Input: dimensioned drawing with shaded views. Units: mm. Origin: part minimum x, y, z. Give positions to 0.01 mm unless a question says otherwise; leave off trailing zeros. Write each loop counter-clockwise with the first axis right and the second up, starting at its lowest first coordinate (ties: lowest second). Pieces come first, ordered by that corner, then holes. Notation, with made-up numbers: M -37,-12.75 L -4,-12.75 A25 ccw -4,26.25 Z; hole C 18,2 d9. An arc over 180 degrees is marked long. Answer as a JSON object with one key per item and string values.
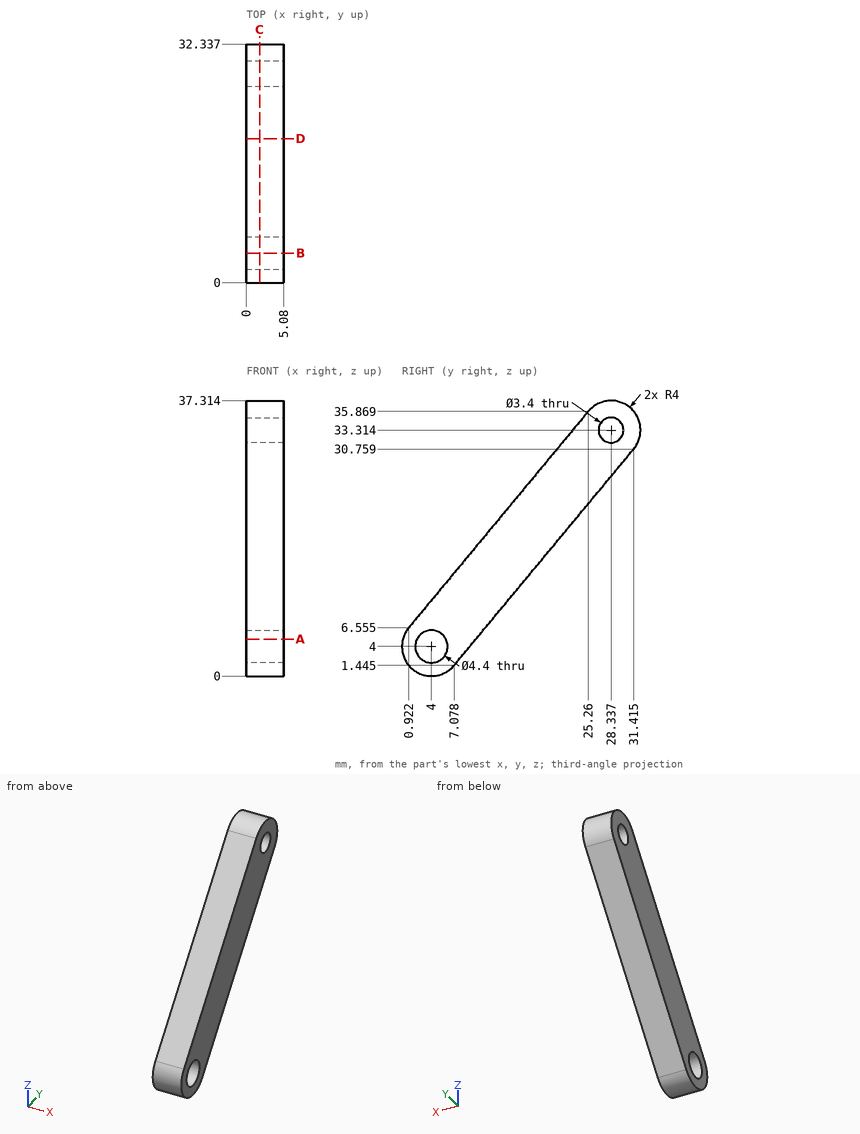
1) Cut plane C-C on x = 1.8. Return loops of the section in (y, z) (1 decimal).
Geometry check:
{"outline": "M 0.9,6.6 A4 ccw 7.1,1.4 L 31.4,30.8 A4 ccw 25.3,35.9 Z; hole C 4,4 d4.4; hole C 28.3,33.3 d3.4"}
2) Cut plane B-B on y = 4. Return loops of the section in (x, z).
Geometry check:
{"outline": "M 0,0 L 5.08,0 L 5.08,1.8 L 0,1.8 Z; M 0,6.2 L 5.08,6.2 L 5.08,10.26 L 0,10.26 Z"}
3) Contact query for flat-ended pins moving along their axis: P1, Ø1.5, axis at x = 3, z = 7, coming from the +Y side; P2, Ø2, axis at x = 3.5, y = 22.5, coming from the -Z side (1 decimal); P3, Ø3, axis at x = 3, y = 26.5, coming from the -Z side. Output: stop coordinate, or through.
Geometry check:
{"P1": "stops at y = 12.31", "P2": "stops at z = 18.8", "P3": "stops at z = 23.03"}
4) Line query: line 1 (Y direction, x = 2.5, z = 4); line 2 (Y direction, x = 3, z = 6) (1 decimal); line 3 (Z direction, x = 2.75, y = 25.5) (1 decimal). Output: solid intervals per line, ascending. Write a range as from..to.
Geometry check:
{"line 1": "y = 0..1.8, 6.2..9.2", "line 2": "y = 0.5..3.1, 4.9..10.9", "line 3": "z = 23.6..36.1"}
5) Cut plane A-A on z = 5. Return loops of the section in (x, y), and give its area (3 significant figures).
Geometry check:
{"outline": "M 0,0.13 L 5.08,0.13 L 5.08,2.04 L 0,2.04 Z; M 0,5.96 L 5.08,5.96 L 5.08,10.03 L 0,10.03 Z", "area": "30.4 mm2"}
6) Cut plane D-D on y = 19.5. Return loops of the section in (x, z).
Geometry check:
{"outline": "M 0,16.41 L 5.08,16.41 L 5.08,28.93 L 0,28.93 Z"}
